from build123d import *

# Parameters (mm, degrees)
SKETCH1_R                   = 3.5
BOSS_EXTRUDE1_DEPTH         = 12
SKETCH3_R                   = 17
BOSS_EXTRUDE2_DEPTH         = 8
FILLET1_R                   = 1.25
CUT_EXTRUDE1_DEPTH          = 36.902646142
CUT_EXTRUDE1_DEPTH_BACK     = 36.902646142
SKETCH4_R                   = 10
CUT_EXTRUDE2_DEPTH          = 40.306488113
CUT_EXTRUDE2_DEPTH_BACK     = 40.306488113
SKETCH5_W                   = 2
SKETCH5_H                   = 20
CUT_EXTRUDE3_DEPTH          = 40.306488113
CUT_EXTRUDE3_DEPTH_BACK     = 40.306488113
SKETCH7_R                   = 3
CUT_EXTRUDE4_DEPTH          = 12.5
FILLET2_R                   = 3
FILLET3_R                   = 1
M5_TAPPED_HOLE2_D           = 4.2
M5_TAPPED_HOLE2_CSINK_D     = 5.05
M5_TAPPED_HOLE2_CSINK_ANGLE = 90
SKETCH26_R                  = 2.5
BOSS_EXTRUDE4_DEPTH         = 0.001
BOSS_EXTRUDE4_DEPTH_BACK    = 25.5
SKETCH28_R                  = 4
BOSS_EXTRUDE5_DEPTH         = 5
CHAMFER1_SIZE               = 0.125
CUT_EXTRUDE5_DEPTH          = 3
FILLET4_R                   = 0.75


with BuildPart() as part:
    # Sketch1 → Boss-Extrude1 (new body)
    with BuildSketch(Plane(origin=(0, 0, 0), x_dir=(1, 0, 0), z_dir=(0, 1, 0))):
        with BuildLine():
            Line((5, -19), (-5, -19))
            Line((-5, -19), (-25.659364193, -4.502045968))
            ThreePointArc((-25.659364193, -4.502045968), (-27.968143757, -0.591103926), (-26.548475243, 3.722881707))
            Line((-26.548475243, 3.722881707), (-12.5, 19))
            Line((-12.5, 19), (12.5, 19))
            Line((12.5, 19), (26.548475243, 3.722881707))
            ThreePointArc((26.548475243, 3.722881707), (27.968143757, -0.591103926), (25.659364193, -4.502045968))
            Line((25.659364193, -4.502045968), (5, -19))
        make_face()
        with Locations(Location((-22.5, 0, 0), (0, 0, 270))):
            Circle(SKETCH1_R, mode=Mode.SUBTRACT)
        with Locations(Location((22.5, 0, 0), (0, 0, 90))):
            Circle(SKETCH1_R, mode=Mode.SUBTRACT)
    extrude(amount=BOSS_EXTRUDE1_DEPTH)

    # Sketch3 → Boss-Extrude2 (add)
    with BuildSketch(Plane(origin=(0, 12, 0), x_dir=(1, 0, 0), z_dir=(0, 1, 0))):
        with Locations(Location((0, 0, 0), (0, 0, 270))):
            Circle(SKETCH3_R)
    extrude(amount=BOSS_EXTRUDE2_DEPTH)

    # Fillet1
    fillet1_edges = [part.edges().sort_by_distance(p)[0] for p in [
        (0, 20, -17),
    ]]
    fillet(fillet1_edges, radius=FILLET1_R)

    # Sketch2 → Cut-Extrude1 (cut, two sides)
    with BuildSketch(Plane(origin=(0, 12, 0), x_dir=(1, 0, 0), z_dir=(0, 1, 0))) as cut_extrude1_sk:
        Polygon((12.5, 19), (12.5, 11), (26.548475243, 3.722881707), align=None)
        Polygon((-12.5, 19), (-12.5, 8.999645995), (-26.548475243, 3.722881707), align=None)
    extrude(amount=CUT_EXTRUDE1_DEPTH, mode=Mode.SUBTRACT)
    extrude(cut_extrude1_sk.sketch, amount=-CUT_EXTRUDE1_DEPTH_BACK, mode=Mode.SUBTRACT)

    # Sketch4 → Cut-Extrude2 (cut, two sides)
    with BuildSketch(Plane(origin=(0, 20, 0), x_dir=(1, 0, 0), z_dir=(0, 1, 0))) as cut_extrude2_sk:
        with Locations(Location((0, 0, 0), (0, 0, 270))):
            Circle(SKETCH4_R)
    extrude(amount=CUT_EXTRUDE2_DEPTH, mode=Mode.SUBTRACT)
    extrude(cut_extrude2_sk.sketch, amount=-CUT_EXTRUDE2_DEPTH_BACK, mode=Mode.SUBTRACT)

    # Sketch5 → Cut-Extrude3 (cut, two sides)
    with BuildSketch(Plane(origin=(0, 20, 0), x_dir=(1, 0, 0), z_dir=(0, 1, 0))) as cut_extrude3_sk:
        with Locations((0, 10)):
            Rectangle(SKETCH5_W, SKETCH5_H)
    extrude(amount=CUT_EXTRUDE3_DEPTH, mode=Mode.SUBTRACT)
    extrude(cut_extrude3_sk.sketch, amount=-CUT_EXTRUDE3_DEPTH_BACK, mode=Mode.SUBTRACT)

    # Sketch7 → Cut-Extrude4 (cut)
    with BuildSketch(Plane.ZY.offset(12.5)):
        with Locations((-15, 6)):
            Circle(SKETCH7_R)
    extrude(amount=-CUT_EXTRUDE4_DEPTH, mode=Mode.SUBTRACT)

    # Fillet2
    fillet2_edges = [part.edges().sort_by_distance(p)[0] for p in [
        (26.548475243, 6, -3.722881707),
        (-26.548475243, 6, -3.722881707),
    ]]
    fillet(fillet2_edges, radius=FILLET2_R)

    # Fillet3
    fillet3_edges = [part.edges().sort_by_distance(p)[0] for p in [
        (5, 6, 19),
        (-5, 6, 19),
    ]]
    fillet(fillet3_edges, radius=FILLET3_R)

    # M5 Tapped Hole2 (through all)
    with Locations(Plane(origin=(12.5, 0, 0), x_dir=(0, 0, -1), z_dir=(1, 0, 0))):
        with Locations((15, 6)):
            CounterSinkHole(M5_TAPPED_HOLE2_D / 2, M5_TAPPED_HOLE2_CSINK_D / 2, counter_sink_angle=M5_TAPPED_HOLE2_CSINK_ANGLE)



with BuildPart() as body_2:
    # Sketch26 → Boss-Extrude4 (new, two sides)
    with BuildSketch(Plane.ZY.offset(12.7)) as boss_extrude4_sk:
        with Locations((-15, 6)):
            Circle(SKETCH26_R)
    extrude(amount=BOSS_EXTRUDE4_DEPTH)
    extrude(boss_extrude4_sk.sketch, amount=-BOSS_EXTRUDE4_DEPTH_BACK)


with BuildPart() as part_1:
    add(part.part)

    add(body_2.part)  # Boss-Extrude5 merges body 2
    # Sketch28 → Boss-Extrude5 (add)
    with BuildSketch(Plane.ZY.offset(12.701)):
        with Locations((-15, 6)):
            Circle(SKETCH28_R)
    extrude(amount=BOSS_EXTRUDE5_DEPTH)

    # Chamfer1
    chamfer1_edges = [part_1.edges().sort_by_distance(p)[0] for p in [
        (12.8, 6, -17.5),
    ]]
    chamfer(chamfer1_edges, length=CHAMFER1_SIZE)

    # Sketch29 → Cut-Extrude5 (cut)
    with BuildSketch(Plane.ZY.offset(17.701)):
        Polygon((-15, 8.309401077), (-17, 7.154700538), (-17, 4.845299462), (-15, 3.690598923), (-13, 4.845299462), (-13, 7.154700538), align=None)
    extrude(amount=-CUT_EXTRUDE5_DEPTH, mode=Mode.SUBTRACT)

    # Fillet4
    fillet4_edges = [part_1.edges().sort_by_distance(p)[0] for p in [
        (-17.701, 6, -19),
    ]]
    fillet(fillet4_edges, radius=FILLET4_R)


solid = part_1.part
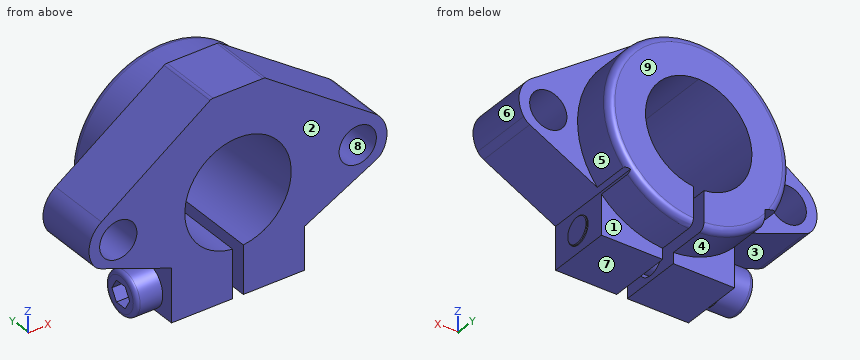
Here's how the part is built. I have some questions about the finished solid (model axes, mm). Face numbers are marked on the shaded views. A direction names the side the tool comes from. Coordinates: 2 decimals unless noted, no trailing zeros. Loops run counter-clockwise (first coordinate to the right, second up) from the corner with the lowest first, then second, coordinate; pieces in that order, holes last.
1. Imagine slicing it at A-A, the plane z = 0. Please give me the cut outline in (x, y), and give its area (3 significant figures).
2. Imagine slicing it at C-C, the plane y = 6. Count the separate pieces of the cut face and the enclosed holes in it, and give its area (3 significant figures).
3. If we mould it in two halves opening along Z, with no side actions, what happens to the marked faces 6, 7, 8 and 9? For each: pulls with the +Z half, pulls with the -Z half, needs draft (parallel to the pull), parting line crosses it, or undercut.
4. Imagine slicing it at D-D, the plane y = 16.25. Please give me the cut outline in (x, z), and give its area (3 significant figures).
5. Imagine slicing it at B-B, the plane x = 24. Please give me the cut outline in (y, z), and give its area (3 significant figures).
6. For P1, Ø4, axis at x = -22.5, z = 0, coming from the -Y side; P2, Ø5, axis at y = 10.5, z = 10, coming from the +X side; P3, Ø9, axis at x = 22.5, z = 0, coming from the -Y side; P4, Ø3.5, axis at y = 6, z = -15, coming from the -X side, each with a flat end and sliding along its axis, tell me the tip position at first contact or that it passes through.
7. For the marked faces 1, 2, 3, 4 and 5, which set-ups out of +Z, -Z, +X, -X, +Y, -Y let a thin tool reach every point of the face, with its end or its side?
8. I need wall thicknesses on L1, parallel to X at y = 8.5, z = 0; L2, parallel to Y at x = -4, z = -15; L3, parallel to Z at x = -21, y = 4.75. Which ranges of each line are inside material? Lowest first, please.
Taken from the geometry:
1. outline: (-28, 0) - (-26, 0) - (-26, 12) - (-28, 12) - close; (-19, 0) - (-10, 0) - (-10, 20) - (-15.75, 20) arc R1.25 ccw to (-17, 18.75) - (-17, 12) - (-19, 12) - close; (10, 0) - (19, 0) - (19, 12) - (17, 12) - (17, 18.75) arc R1.25 ccw to (15.75, 20) - (10, 20) - close; (26, 0) - (28, 0) - (28, 12) - (26, 12) - close
1. area: 375 mm2
2. separate pieces: 2
2. enclosed holes: 2
2. area: 985 mm2
3. face 6: parting line crosses it
3. face 7: pulls with the -Z half
3. face 8: undercut
3. face 9: needs draft
4. outline: (-14.96, -8.08) - (-12.5, -9) - (-12.5, -11.52) arc R17 ccw to (-1, -16.97) - (-1, -9.95) arc R10 cw (long way) to (1, -9.95) - (1, -16.97) arc R17 ccw to (12.5, -11.52) - (12.5, -11) - (13.3, -10.58) arc R17 ccw (long way) to start
4. area: 576 mm2
5. outline: (0, -5.04) - (12, -5.04) - (12, -3.16) - (0, -3.16) - close; (0, 3.16) - (12, 3.16) - (12, 5.67) - (0, 5.67) - close
5. area: 52.6 mm2
6. P1: passes through
6. P2: stops at x = 21.39
6. P3: stops at y = 0
6. P4: stops at x = -14.7
7. face 1: -Z, +X, +Y
7. face 2: +Z, -Z, +X, -X, -Y
7. face 3: -X, +Y, -Y
7. face 4: -Z, -X, +Y
7. face 5: +Y
8. L1: x = -28 to -26, -19 to -10, 10 to 19, 26 to 28
8. L2: y = 0 to 3, 3.5 to 8.5, 9 to 20
8. L3: z = -5.81 to -3.16, 3.16 to 7.77
